The model under review builds one solid part; all positions refer to its coordinate system, in mm. Give positions to 0.01 mm unless a question says otherwise; leave off trailing zeros. Order: outer loops, then holes, each group sorted by start corner. A loop starts at its lowest first (then second) coordinate and runs counter-clockwise, first axis right, second up. Notation, with made-up numbers: (39, 75) -> (95, 75) arc R12 ccw to (95, 85) -> close; hole circle Ø9 at (63.25, -5). An arc over 180 degrees is marked (long way). Answer as a JSON object with one key per item and string values. Group by question number.
from build123d import *

# Parameters (mm, degrees)
BOSS_EXTRUDE1_DEPTH = 25.4
CHAMFER1_SIZE       = 25.4


with BuildPart() as part:
    # Sketch2 → Boss-Extrude1 (new body)
    with BuildSketch(Plane.XY):
        with BuildLine():
            Line((-28.394744795, 6.35), (-101.6, 6.35))
            Line((-101.6, 6.35), (-101.6, 50.8))
            Line((-101.6, 50.8), (-67.239627541, 50.8))
            ThreePointArc((-67.239627541, 50.8), (-49.99007984, 26.676106864), (-28.394744795, 6.35))
        make_face()
    extrude(amount=-BOSS_EXTRUDE1_DEPTH)

    # Chamfer1
    chamfer1_edges = [part.edges().sort_by_distance(p)[0] for p in [
        (-101.6, 50.8, -12.7),
    ]]
    chamfer(chamfer1_edges, length=CHAMFER1_SIZE)


solid = part.part
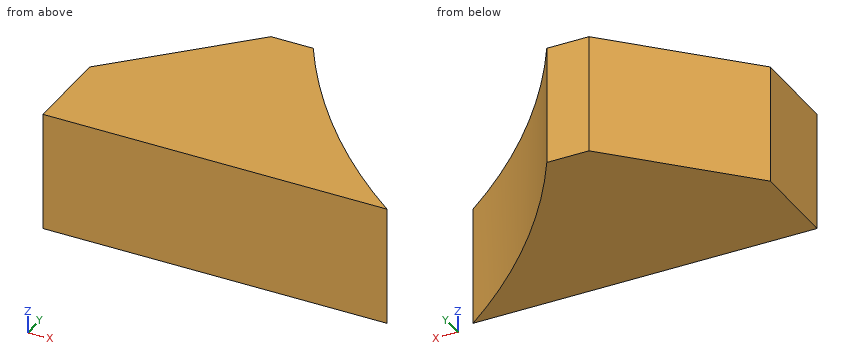
1. Take a section at B-B on x = -85. Give the boundary of the cut face in (y, z), plus the area to 3 significant figures.
2. Take a section at A-A on z = -19.5. Give the boundary of the cut face in (x, y), plus the area to 3 significant figures.
3. For probe 1 along X at (y, z) = (19.5, -19.5); probe 2 along Y at (x, z) = (-46, -21.75); probe 3 along Y at (x, z) = (-63, -18.25), list the stretches that pass through material, from the lowest coordinate up. Write a range as [from, to].
4. For pin 1 (3 mm diameter, centred on x = -37.5, y = 17.5, fed in from -Z); pin 2 (1.5 mm diameter, centred on y = 38, z = -9.5, fed in from -X); pin 3 (8 mm diameter, centred on x = -82, z = -22.5, fed in from +Y); pin 4 (1 mm diameter, centred on y = 34.5, z = -15, fed in from -X), all flat-tipped, find the tip position at first contact; note any pin that passes through.
5. Take a section at C-C on y = 42.5. Give the boundary of the cut face in (x, z).
Checks:
{
 "1": {"outline": "(6.35, -25.4) -> (42, -25.4) -> (42, 0) -> (6.35, 0) -> close", "area": "906 mm2"},
 "2": {"outline": "(-101.6, 6.35) -> (-28.39, 6.35) arc R152.39 cw to (-67.24, 50.8) -> (-76.2, 50.8) -> (-101.6, 25.4) -> close", "area": "1,950 mm2"},
 "3": {"probe 1": "x = [-101.6, -43.3]", "probe 2": "y = [6.35, 22.29]", "probe 3": "y = [6.35, 43.88]"},
 "4": {"pin 1": "passes through", "pin 2": "stops at x = -89.75", "pin 3": "stops at y = 49", "pin 4": "stops at x = -93"},
 "5": {"outline": "(-84.5, -25.4) -> (-62.09, -25.4) -> (-62.09, 0) -> (-84.5, 0) -> close"}
}
